Check sheet for the modelled part. Datum: model origin and axes. Units: mm. Give positions to 0.01 mm unless a question says otherwise; leave off trailing zeros. Loops run counter-clockwise (first coordinate to the right, second up) from the corner with the lowest first, then second, coordinate; pieces in that order, holes last. Notation, with made-up numbers: (79, -21) -> (95, -21) arc R20 cw to (95, -6) -> close; hole circle Ø9 at (28.5, -3). An arc over 180 degrees is marked (long way). Answer as CSV lines item,"result". Start each with the question number.
(1) Section check A-A on y = -20.5. Enter the section's corners in (x, z).
(2) Material ranges on line 1 (X direction, y = -88, z = 0.75); line 2 (X direction, y = 92.5, z = 2); line 3 (Y direction, x = -68, z = 1.5), recorded low to high. Write a range as from..to.
(3) Section check B-B on z = 4.5. State how many separate pieces and enclosed holes the cut face has, plus the area to 3 significant figures.
from build123d import *

# Parameters (mm, degrees)
SKETCH1_W                   = 105.470303733
SKETCH1_H                   = 273.610686589
SKETCH1_R                   = 3
BOSS_EXTRUDE2_DEPTH         = 6.35
CUTOUT_FILLETS_R            = 5
CUTOUT_FILLETS_OF_MIRROR2_R = 5


with BuildPart() as part:
    # Sketch1 → Boss-Extrude2 (new body)
    with BuildSketch(Plane.XY):
        with Locations((52.735151867, 0.297634424)):
            Rectangle(SKETCH1_W, SKETCH1_H)
        with Locations((29.45532979, -128.937258766)):
            Circle(SKETCH1_R, mode=Mode.SUBTRACT)
        with Locations((76.788897449, -128.937258766)):
            Circle(SKETCH1_R, mode=Mode.SUBTRACT)
        with Locations((97.306985108, 119.786891803)):
            Circle(SKETCH1_R, mode=Mode.SUBTRACT)
        with Locations((97.306985108, -0.213108197)):
            Circle(SKETCH1_R, mode=Mode.SUBTRACT)
        with Locations((97.306985108, -112.213108197)):
            Circle(SKETCH1_R, mode=Mode.SUBTRACT)
        Polygon((4, 119.786891803), (4, 71.260960171), (76.788897449, 119.786891803), align=None, mode=Mode.SUBTRACT)
        Polygon((86, 116.312823436), (13.211102551, 67.786891803), (86, 67.786891803), align=None, mode=Mode.SUBTRACT)
        Polygon((13.211102551, 59.786891803), (86, 59.786891803), (86, 11.260960171), align=None, mode=Mode.SUBTRACT)
        Polygon((76.788897449, 7.786891803), (4, 56.312823436), (4, 7.786891803), align=None, mode=Mode.SUBTRACT)
        Polygon((4, -0.213108197), (76.788897449, -0.213108197), (4, -48.739039829), align=None, mode=Mode.SUBTRACT)
        Polygon((86, -3.687176564), (13.211102551, -52.213108197), (86, -52.213108197), align=None, mode=Mode.SUBTRACT)
        Polygon((13.211102551, -60.213108197), (86, -60.213108197), (86, -108.739039829), align=None, mode=Mode.SUBTRACT)
        Polygon((4, -112.213108197), (4, -63.687176564), (76.788897449, -112.213108197), align=None, mode=Mode.SUBTRACT)
    boss_extrude2 = extrude(amount=BOSS_EXTRUDE2_DEPTH)

    # Cutout_Fillets
    cutout_fillets_edges = [part.edges().sort_by_distance(p)[0] for p in [
        (76.788897449, 119.786891803, 3.175),
        (4, 119.786891803, 3.175),
        (4, 71.260960171, 3.175),
        (86, 67.786891803, 3.175),
        (86, 116.312823436, 3.175),
        (13.211102551, 67.786891803, 3.175),
        (13.211102551, 59.786891803, 3.175),
        (86, 11.260960171, 3.175),
        (86, 59.786891803, 3.175),
        (4, 7.786891803, 3.175),
        (76.788897449, 7.786891803, 3.175),
        (4, 56.312823436, 3.175),
        (4, -0.213108197, 3.175),
        (4, -48.739039829, 3.175),
        (76.788897449, -0.213108197, 3.175),
        (86, -52.213108197, 3.175),
        (86, -3.687176564, 3.175),
        (13.211102551, -52.213108197, 3.175),
        (13.211102551, -60.213108197, 3.175),
        (86, -108.739039829, 3.175),
        (86, -60.213108197, 3.175),
        (4, -112.213108197, 3.175),
        (76.788897449, -112.213108197, 3.175),
        (4, -63.687176564, 3.175),
    ]]
    fillet(cutout_fillets_edges, radius=CUTOUT_FILLETS_R)

    # Mirror2: Boss-Extrude2 across plane
    add(boss_extrude2.mirror(Plane(origin=(0, 137.102977719, 6.35), x_dir=(0, 0, 1), z_dir=(1, 0, 0))))

    # Cutout_Fillets of Mirror2
    cutout_fillets_of_mirror2_edges = [part.edges().sort_by_distance(p)[0] for p in [
        (-76.788897449, 119.786891803, 3.175),
        (-4, 119.786891803, 3.175),
        (-4, 71.260960171, 3.175),
        (-86, 67.786891803, 3.175),
        (-86, 116.312823436, 3.175),
        (-13.211102551, 67.786891803, 3.175),
        (-13.211102551, 59.786891803, 3.175),
        (-86, 11.260960171, 3.175),
        (-86, 59.786891803, 3.175),
        (-4, 7.786891803, 3.175),
        (-76.788897449, 7.786891803, 3.175),
        (-4, 56.312823436, 3.175),
        (-4, -0.213108197, 3.175),
        (-4, -48.739039829, 3.175),
        (-76.788897449, -0.213108197, 3.175),
        (-86, -52.213108197, 3.175),
        (-86, -3.687176564, 3.175),
        (-13.211102551, -52.213108197, 3.175),
        (-13.211102551, -60.213108197, 3.175),
        (-86, -108.739039829, 3.175),
        (-86, -60.213108197, 3.175),
        (-4, -112.213108197, 3.175),
        (-76.788897449, -112.213108197, 3.175),
        (-4, -63.687176564, 3.175),
    ]]
    fillet(cutout_fillets_of_mirror2_edges, radius=CUTOUT_FILLETS_OF_MIRROR2_R)


solid = part.part
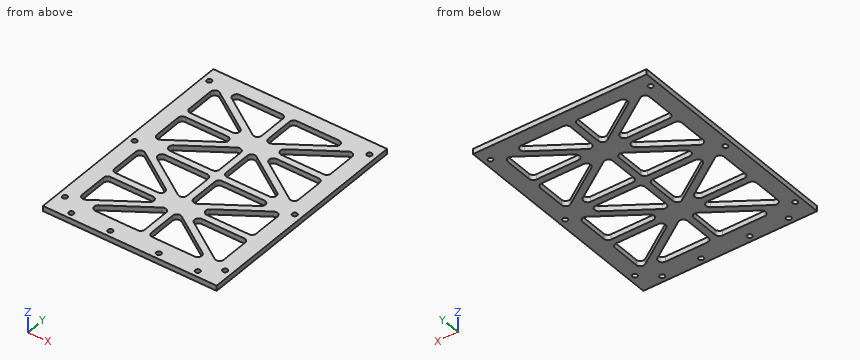
Working result:
1,outline,"(-105.47, 0) -> (-86, 0) -> (-86, 6.35) -> (-105.47, 6.35) -> close; (-60.78, 0) -> (-46.36, 0) -> (-46.36, 6.35) -> (-60.78, 6.35) -> close; (-4, 0) -> (4, 0) -> (4, 6.35) -> (-4, 6.35) -> close; (46.36, 0) -> (60.78, 0) -> (60.78, 6.35) -> (46.36, 6.35) -> close; (86, 0) -> (105.47, 0) -> (105.47, 6.35) -> (86, 6.35) -> close"
2,line 1,"x = -105.47..-86, -54.89..-40.47, -4..4, 40.47..54.89, 86..105.47"
2,line 2,"x = -105.47..-86, -50.28..-35.86, -4..4, 35.86..50.28, 86..105.47"
2,line 3,"y = -136.51..-96.74, -60.21..-52.21, -15.69..23.26, 59.79..67.79, 104.31..137.1"
3,separate pieces,"1"
3,enclosed holes,"26"
3,area,"30,400 mm^2"
